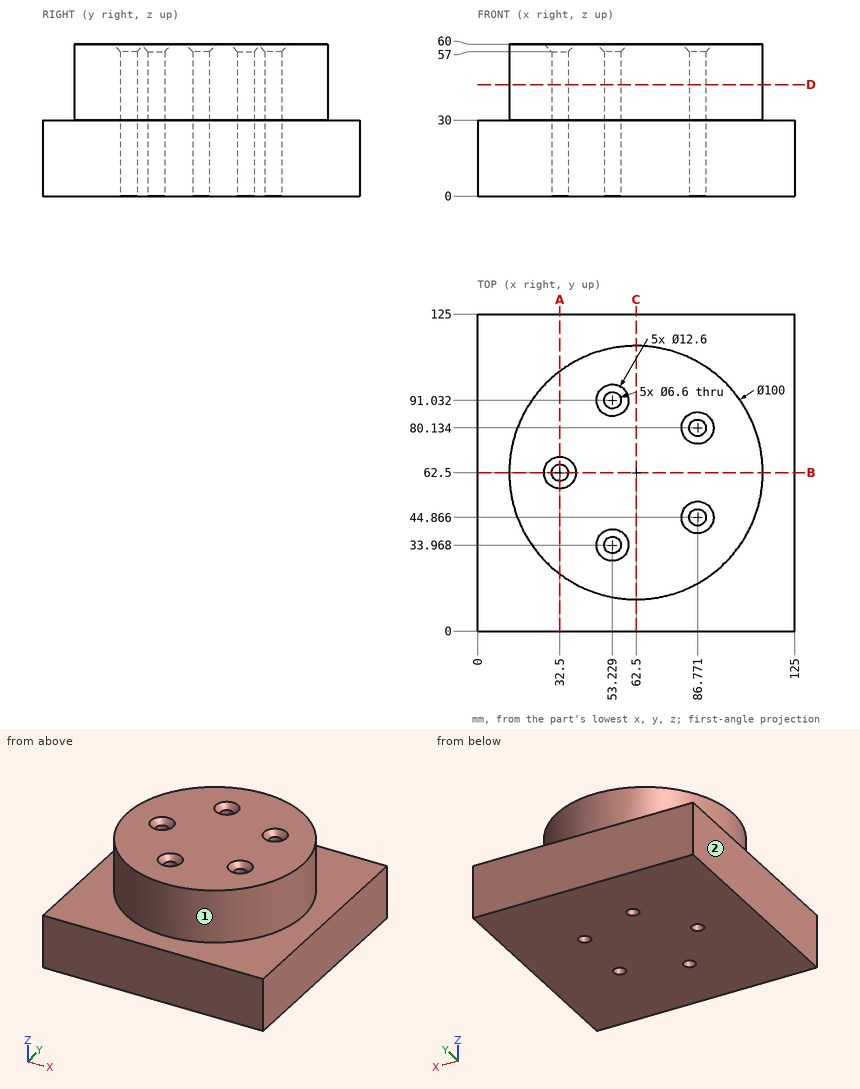
For this review, use the dimensioned drawing (mm, ordinates from the lowest corner) and the shaded views. A direction names the side the tool comes from. Coordinates: 2 decimals unless noted, no trailing zeros. Order: outer loops, then holes, each group sorted by start corner. A loop starts at its lowest first (then second) coordinate and runs counter-clockwise, first axis right, second up. Notation, with made-up numbers: (-37, 24.5) -> (-14, 24.5) arc R12 cw to (-14, 30.5) -> close; hole circle Ø6 at (18, -17). An arc over 180 degrees is marked (long way). One line per item, written item: value. Start each with the question number.
Q1. Take a section at D-D, the plane z = 44. State the section outline as (x, y) points, then the cut area to 3 significant figures.
Q2. Take a section at A-A, the plane x = 32.5. State the section outline as (y, z) points.
Q3. Take a section at B-B, the plane y = 62.5. State the section outline as (x, z) points, then the cut area to 4 significant figures.
Q4. Take a section at C-C, the plane x = 62.5. State the section outline as (y, z) points, then the cut area to 3 significant figures.
Q5. For probe 1 along Y at (x, z) = (53, 16); probe 2 along Y at (x, z) = (88, 40.5) (1 decimal); probe 3 along Z at (x, y) = (97, 11), list the stretches that pass through material, from the lowest coordinate up.
Q6. Insertion check: pin 1 Ø4 at (x, z) = (93.5, 15) entering from -Y; pin 2 Ø6 at (x, y) = (86.77, 80.13) entering from -Z; pin 3 Ø6 at (x, z) = (44, 43.5) entering from -Y; pin 4 Ø5 at (x, z) = (14.5, 46.5) entering from -Y. Each pin has a flat end and moves straight along its axis. Give the tip position at first contact, or say it passes through.
Q7. Tool access review of the marked faces 1 and 2: name each direction out of +Z, -Z, +X, -X, +Y, -Y from which nothing blocks a thin tool from reaching the whole face with its end or side.
Values follow:
1. outline: circle Ø100 at (62.5, 62.5); hole circle Ø6.6 at (32.5, 62.5); hole circle Ø6.6 at (53.23, 33.97); hole circle Ø6.6 at (53.23, 91.03); hole circle Ø6.6 at (86.77, 44.87); hole circle Ø6.6 at (86.77, 80.13)
1. area: 7,680 mm2
2. outline: (0, 0) -> (59.2, 0) -> (59.2, 57) -> (56.2, 60) -> (22.5, 60) -> (22.5, 30) -> (0, 30) -> close; (65.8, 0) -> (125, 0) -> (125, 30) -> (102.5, 30) -> (102.5, 60) -> (68.8, 60) -> (65.8, 57) -> close
3. outline: (0, 0) -> (29.2, 0) -> (29.2, 57) -> (26.2, 60) -> (12.5, 60) -> (12.5, 30) -> (0, 30) -> close; (35.8, 0) -> (125, 0) -> (125, 30) -> (112.5, 30) -> (112.5, 60) -> (38.8, 60) -> (35.8, 57) -> close
3. area: 6,345 mm2
4. outline: (0, 0) -> (125, 0) -> (125, 30) -> (112.5, 30) -> (112.5, 60) -> (12.5, 60) -> (12.5, 30) -> (0, 30) -> close
4. area: 6,750 mm2
5. probe 1: y = 0 to 30.68, 37.26 to 87.74, 94.32 to 125
5. probe 2: y = 19.5 to 41.8, 47.9 to 77.1, 83.2 to 105.5
5. probe 3: z = 0 to 30
6. pin 1: stops at y = 0
6. pin 2: passes through
6. pin 3: stops at y = 14.96
6. pin 4: stops at y = 41.77
7. face 1: +Z
7. face 2: +Z, -Z, -X, +Y, -Y
